The model under review builds one solid part; all positions refer to its coordinate system, in mm. A direction names the side the tool comes from. Round coordinates to 2 decimals unless told otherwise and drop trailing zeros. Write each loop counter-clockwise with the first axis right and the second up, starting at its lowest first coordinate (ties: lowest second). Pieces come first, ordered by that corner, then holes. Notation, with made-up numbers: (26.25, 65.5) -> (69.25, 65.5) arc R17 ccw to (69.25, 84.5) -> close; hole circle Ø8 at (81.5, -15). An arc over 180 degrees is marked (long way). Return JSON: item names as keys, results as strings. Group by question number.
1. Clearance check with a flat-ended pin moving along its axis: P1, Ø6, axis at y = 5.1, z = 0, coming from the -X side. State where the tip first meets the part, or that it passes through.
2. Take a section at A-A, the plane z = 0. Write out the cut boundary in (x, y), then the cut area to 3 significant figures.
3. Take a section at B-B, the plane x = -2. Write out the cut boundary in (y, z).
4. Take a section at C-C, the plane y = 15.5. Write out the cut boundary in (x, z), then the cut area to 3 significant figures.
5. Take a section at D-D, the plane z = 3.75. Write out the cut boundary in (x, y).
6. Tool access review of faces 1 (the flat face through (2, 49, 10)), 2 (the flat face through (-2, 49, 7.5)): name each direction out of +Z, -Z, +X, -X, +Y, -Y from which nothing blocks a thin tool from reaching the whole face with its end or side.
7. Mouldability with a two-part tool opening along Z and no side actions: class faces 3 (the flat face through (10, 49, 0)), 4 (the flat face through (4, 98, 7)), 5 (the cylindrical face through (5.07, 92.595, 1.2)), 6 (the cylindrical face through (5.07, 7.677, -0.338)) as pulls with the +Z half, pulls with the -Z half, needs draft (parallel to the pull), parting line crosses it, or undercut.
8. For line 1 along Y through (x, z) = (8.25, 0); line 2 along Z through (x, y) = (2, 95); line 3 along Z through (x, y) = (-2, 39), list the stretches that pass through material, from the lowest coordinate up. Write a range as from..to.
from build123d import *

# Parameters (mm, degrees)
EXTRUDE_1_DEPTH          = 100
CUT_EXTRUDE_1_DEPTH      = 101.995049384
CUT_EXTRUDE_1_DEPTH_BACK = 101.995049384
SKETCH_2_R               = 2.6


with BuildPart() as part:
    # 草图1 → 凸台-拉伸1 (new body)
    with BuildSketch(Plane(origin=(0, 0, 0), x_dir=(1, 0, 0), z_dir=(0, 1, 0))):
        Polygon((-5, 7.5), (0, 7.5), (0, -7.5), (-5, -7.5), (-5, -10), (10, -10), (10, 10), (-5, 10), align=None)
    extrude(amount=EXTRUDE_1_DEPTH)

    # 草图2 → 切除-拉伸1 (cut, two sides: drawn at the far end of the back side and taken through both)
    with BuildSketch(Plane.ZY.offset(-CUT_EXTRUDE_1_DEPTH_BACK)):
        with Locations((0, 94.901280605)):
            Circle(SKETCH_2_R)
        with Locations((0, 5.098719395)):
            Circle(SKETCH_2_R)
        Polygon((-5, 100), (-10, 95), (-10, 100), align=None)
        Polygon((10, 100), (5, 100), (10, 95), align=None)
        Polygon((-10, 0), (-5, 0), (-10, 5), align=None)
        Polygon((10, 5), (10, 0), (5, 0), align=None)
    extrude(amount=CUT_EXTRUDE_1_DEPTH + CUT_EXTRUDE_1_DEPTH_BACK, mode=Mode.SUBTRACT)


solid = part.part
Output:
{
 "1": {"P1": "stops at x = 0"},
 "2": {"outline": "(0, 0) -> (10, 0) -> (10, 2.5) -> (0, 2.5) -> close; (0, 7.7) -> (10, 7.7) -> (10, 92.3) -> (0, 92.3) -> close; (0, 97.5) -> (10, 97.5) -> (10, 100) -> (0, 100) -> close", "area": "896 mm^2"},
 "3": {"outline": "(2.5, -7.5) -> (5, -10) -> (95, -10) -> (97.5, -7.5) -> close; (2.5, 7.5) -> (97.5, 7.5) -> (95, 10) -> (5, 10) -> close"},
 "4": {"outline": "(-5, -10) -> (10, -10) -> (10, 10) -> (-5, 10) -> (-5, 7.5) -> (0, 7.5) -> (0, -7.5) -> (-5, -7.5) -> close", "area": "225 mm^2"},
 "5": {"outline": "(0, 0) -> (10, 0) -> (10, 100) -> (0, 100) -> close"},
 "6": {"face 1": "+Z, +X, -X, +Y, -Y", "face 2": "-X, +Y, -Y"},
 "7": {"face 3": "needs draft", "face 4": "pulls with the +Z half", "face 5": "undercut", "face 6": "undercut"},
 "8": {"line 1": "y = 0..2.5, 7.7..92.3, 97.5..100", "line 2": "z = -10..-2.6, 2.6..10", "line 3": "z = -10..-7.5, 7.5..10"}
}
